Work out the finished part from the listing and answer in its coordinate system (mm). Face numbers are marked on the shaded views. Round coordinates to 2 decimals unless told otherwise and drop trailing zeros. Loops run counter-clockwise (first coordinate to the right, second up) from the corner with the lowest first, then second, coordinate; pieces in that order, holes last.
```python
from build123d import *

# Parameters (mm, degrees)
SALIENTE_EXTRUIR1_DEPTH = 7.5
CROQUIS2_R              = 1.5
CORTAR_EXTRUIR1_DEPTH   = 147.100350787
REDONDEO1_R             = 3
REDONDEO2_R             = 3
CORTAR_EXTRUIR3_DEPTH   = 161.092886788
CROQUIS5_R              = 2.25
CORTAR_EXTRUIR4_DEPTH   = 133.941951618
CORTAR_EXTRUIR5_DEPTH   = 161.092886788
CROQUIS7_R              = 2.25
CORTAR_EXTRUIR6_DEPTH   = 7
REDONDEO3_R             = 5


with BuildPart() as part:
    # Croquis1 → Saliente-Extruir1 (new, symmetric)
    with BuildSketch(Plane.XY):
        Polygon((0, -3.5), (0, 3.5), (20, 3.5), (20, 5.5), (-100.18, 5.5), (-100.18, 85.5), (-85.18, 85.5), (-85.18, 105.5), (-106.25, 105.5), (-106.25, -5.5), (20, -5.5), (20, -3.5), align=None)
    extrude(amount=SALIENTE_EXTRUIR1_DEPTH, both=True)

    # Croquis2 → Cortar-Extruir1 (cut, through all)
    with BuildSketch(Plane(origin=(0, 5.5, 0), x_dir=(1, 0, 0), z_dir=(0, 1, 0))):
        with Locations(Location((15, 0, 0), (0, 0, 180))):
            Circle(CROQUIS2_R)
        with Locations(Location((5, 0, 0), (0, 0, 180))):
            Circle(CROQUIS2_R)
    extrude(amount=-CORTAR_EXTRUIR1_DEPTH, mode=Mode.SUBTRACT)

    # Redondeo1
    redondeo1_edges = [part.edges().sort_by_distance(p)[0] for p in [
        (20, -4.5, -7.5),
        (20, 4.5, -7.5),
        (20, 4.5, 7.5),
        (20, -4.5, 7.5),
    ]]
    fillet(redondeo1_edges, radius=REDONDEO1_R)

    # Redondeo2
    redondeo2_edges = [part.edges().sort_by_distance(p)[0] for p in [
        (-85.18, 95.5, -7.5),
        (-85.18, 95.5, 7.5),
    ]]
    fillet(redondeo2_edges, radius=REDONDEO2_R)

    # Croquis4 → Cortar-Extruir3 (cut, through all)
    with BuildSketch(Plane(origin=(-100.18, 0, 0), x_dir=(0, 0, -1), z_dir=(1, 0, 0))):
        Polygon((-7.5, 90.5), (7.5, 105.5), (-7.5, 105.5), align=None)
        Polygon((-7.5, 85.5), (7.5, 100.5), (7.5, 85.5), align=None)
    extrude(amount=CORTAR_EXTRUIR3_DEPTH, mode=Mode.SUBTRACT)

    # Croquis5 → Cortar-Extruir4 (cut, through all)
    with BuildSketch(Plane(origin=(0, 49, 49), x_dir=(1, 0, 0), z_dir=(0, 0.7071067811865464, 0.7071067811865488))):
        with Locations(Location((-89.98, 69.296464556, 0), (0, 0, 270))):
            Circle(CROQUIS5_R)
    extrude(amount=-CORTAR_EXTRUIR4_DEPTH, mode=Mode.SUBTRACT)

    # Croquis6 → Cortar-Extruir5 (cut, through all)
    with BuildSketch(Plane(origin=(-100.18, 0, 0), x_dir=(0, 0, -1), z_dir=(1, 0, 0))):
        Polygon((-7.5, 105.5), (-7.5, 90.5), (7.5, 105.5), align=None)
    extrude(amount=-CORTAR_EXTRUIR5_DEPTH, mode=Mode.SUBTRACT)

    # Croquis7 → Cortar-Extruir6 (cut)
    with BuildSketch(Plane(origin=(0, 5.5, 0), x_dir=(1, 0, 0), z_dir=(0, 1, 0))):
        with Locations(Location((-68.75, 0, 0), (0, 0, 180))):
            Circle(CROQUIS7_R)
    extrude(amount=-CORTAR_EXTRUIR6_DEPTH, mode=Mode.SUBTRACT)

    # Redondeo3
    redondeo3_edges = [part.edges().sort_by_distance(p)[0] for p in [
        (-100.18, 93, 0),
        (-106.25, 98, 0),
        (-106.25, -5.5, 0),
        (-100.18, 5.5, 0),
    ]]
    fillet(redondeo3_edges, radius=REDONDEO3_R)


solid = part.part
```
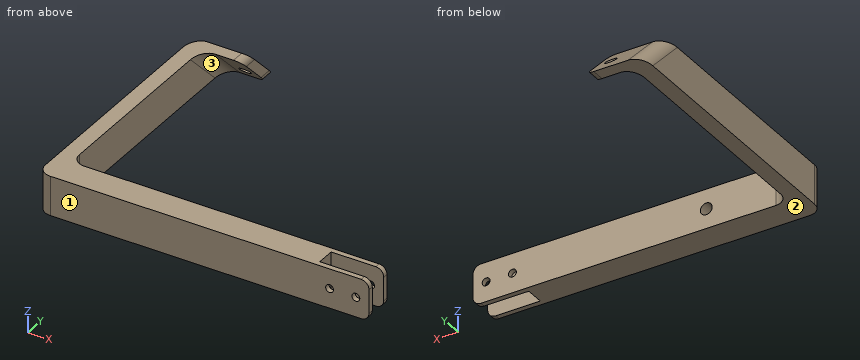
1. Consider probe 1 along Y at (x, z) = (7, 0.5); probe 2 along Z at (x, y) = (5, 4.85); probe 3 along X at (y, z) = (32, 2.5). Determine where each line is inside the solid, lowest interval first.
Answer key:
probe 1: y = -5.5 to -3.5, 3.5 to 5.5
probe 2: z = -7.5 to -1.5, 1.5 to 7.5
probe 3: x = -106.25 to -100.18
2. Determine the mould class of the marked faces 1, 2 and 3 for opening direction Y: +Y half, -Y half, draft (parallel to the pull), parting line (faces both ways), or undercut.
Answer key:
face 1: -Y half
face 2: draft
face 3: undercut
3. Find section A-A (x = 5). Write down the section's boundary in (y, z), then the cut area to 3 significant figures.
Answer key:
outline: (-5.5, -7.5) - (-3.5, -7.5) - (-3.5, -1.5) - (-5.5, -1.5) - close; (-5.5, 1.5) - (-3.5, 1.5) - (-3.5, 7.5) - (-5.5, 7.5) - close; (3.5, -7.5) - (5.5, -7.5) - (5.5, -1.5) - (3.5, -1.5) - close; (3.5, 1.5) - (5.5, 1.5) - (5.5, 7.5) - (3.5, 7.5) - close
area: 48.0 mm2
4. Given pin 1 (3.5 mm diameter, centred on y = -0.5, z = 3, fed in from +X); pin 2 (1.5 mm diameter, centred on y = 83.5, z = 5, fed in from +X); pin 3 (10 mm diameter, centred on x = -10, y = 13.5, fed in from +Z); pin 4 (3.5 mm diameter, centred on x = 15, z = 0, fed in from +Y), each flat-ended and moving along its own axis, determine where each tip first touches the part or whether it passes through.
Answer key:
pin 1: stops at x = 0
pin 2: stops at x = -99.47
pin 3: passes through
pin 4: stops at y = 5.5
5. Find section B-B (x = -68.75). Write down the section's boundary in (y, z).
Answer key:
outline: (-5.5, -7.5) - (5.5, -7.5) - (5.5, -2.25) - (-1.5, -2.25) - (-1.5, 2.25) - (5.5, 2.25) - (5.5, 7.5) - (-5.5, 7.5) - close
6. Find section D-D (x = -18). Write down the section's boundary in (y, z), then the cut area to 3 significant figures.
Answer key:
outline: (-5.5, -7.5) - (5.5, -7.5) - (5.5, 7.5) - (-5.5, 7.5) - close
area: 165 mm2
7. Find section C-C (y = 23.5). Write down the section's boundary in (x, z).
Answer key:
outline: (-106.25, -7.5) - (-100.18, -7.5) - (-100.18, 7.5) - (-106.25, 7.5) - close
